Here's how the part is built. I have some questions about the finished solid (model axes, mm). A direction names the side the tool comes from. Round coordinates to 2 decimals unless told otherwise and drop trailing zeros. Loops run counter-clockwise (first coordinate to the right, second up) from the corner with the lowest first, then second, coordinate; pieces in that order, holes last. Notation, with made-up numbers: M -38,-35 L 5,-35 A6 cw 5,-30 Z; hole C -3,52.25 d8. An arc over 180 degrees is marked long. Answer as a JSON object with one key per item and string values.
from build123d import *

# Parameters (mm, degrees)
SKETCH1_W           = 100
SKETCH1_H           = 99
BOSS_EXTRUDE1_DEPTH = 12.75
SKETCH2_W           = 13
SKETCH2_H           = 10
CUT_EXTRUDE1_DEPTH  = 20
LPATTERN1_COUNT     = 5
LPATTERN1_PITCH     = 16
SKETCH3_R           = 1.5
CUT_EXTRUDE2_DEPTH  = 10


with BuildPart() as part:
    # Sketch1 → Boss-Extrude1 (new, symmetric)
    with BuildSketch(Plane(origin=(0, 0, 0), x_dir=(1, 0, 0), z_dir=(0, 1, 0))):
        Rectangle(SKETCH1_W, SKETCH1_H)
    extrude(amount=BOSS_EXTRUDE1_DEPTH, both=True)

    # Sketch2 → Cut-Extrude1 (cut)
    with BuildSketch(Plane.XY.offset(49.5)):
        with Locations((-37, 0)):
            Rectangle(SKETCH2_W, SKETCH2_H)
    cut_extrude1 = extrude(amount=-CUT_EXTRUDE1_DEPTH, mode=Mode.SUBTRACT)

    # LPattern1: Cut-Extrude1 ×5
    with Locations(*[(i * LPATTERN1_PITCH, 0, 0) for i in range(1, LPATTERN1_COUNT)]):
        add(cut_extrude1, mode=Mode.SUBTRACT)

    # Sketch3 → Cut-Extrude2 (cut)
    with BuildSketch(Plane(origin=(0, 0, -49.5), x_dir=(-1, 0, 0), z_dir=(0, 0, -1))):
        with Locations((29, 0)):
            Circle(SKETCH3_R)
    extrude(amount=-CUT_EXTRUDE2_DEPTH, mode=Mode.SUBTRACT)


solid = part.part
Item 1: On a 3-axis mill with a long thin cutter (end or side, diameter ignored), from which of +Z, -Z, +X, -X, +Y, -Y can I reach the whole of each face in a straight line? I mean faces 4 (the face through (-27.5, 0.07, -44.57)), 5 (the face through (-5, 5, 40)), 6 (the face through (-0.7, -5.5, 49.5)). Say none if no direction works.
Resolved:
{"face 4": "-Z", "face 5": "+Z", "face 6": "+Z, +X, -X, +Y, -Y"}
Item 2: I want a section at B-B, the plane x = -17. Please give me the cut outline in (y, z), then the cut area to 3 significant figures.
Resolved:
{"outline": "M -12.75,-49.5 L 12.75,-49.5 L 12.75,49.5 L 5,49.5 L 5,29.5 L -5,29.5 L -5,49.5 L -12.75,49.5 Z", "area": "2,320 mm²"}
Item 3: I'm going to push a flat-ended pin straight in: pin 1 Ø5 at (x, y) = (28.5, 2) entering from +Z. Where does the tip first touch, or does it pass through?
Resolved:
{"pin 1": "z = 29.5"}
Item 4: Please list where these lines run through material, in increasing order: probe 1 along X at (y, z) = (-4.75, 30.5); probe 2 along Y at (x, z) = (-29, -45); probe 3 along Z at (x, y) = (30, -1.75). Write a range as from..to.
Resolved:
{"probe 1": "-50..-43.5, -30.5..-27.5, -14.5..-11.5, 1.5..4.5, 17.5..20.5, 33.5..50", "probe 2": "-12.75..-1.5, 1.5..12.75", "probe 3": "-49.5..29.5"}
Item 5: I want a section at A-A, the plane y = 3. Please give me the cut outline in (x, z), then the cut area to 3 significant figures.
Resolved:
{"outline": "M -50,-49.5 L 50,-49.5 L 50,49.5 L 33.5,49.5 L 33.5,29.5 L 20.5,29.5 L 20.5,49.5 L 17.5,49.5 L 17.5,29.5 L 4.5,29.5 L 4.5,49.5 L 1.5,49.5 L 1.5,29.5 L -11.5,29.5 L -11.5,49.5 L -14.5,49.5 L -14.5,29.5 L -27.5,29.5 L -27.5,49.5 L -30.5,49.5 L -30.5,29.5 L -43.5,29.5 L -43.5,49.5 L -50,49.5 Z", "area": "8,600 mm²"}
Item 6: If we mould it in two halves opening along X, with no side actions, what happens to faces 1 (the face through (-1, 0, -49.5)), 2 (the face through (-37, -5, 40)), 3 (the face through (50, 0, 1))? For each: pulls with the +X half, pulls with the -X half, needs draft (parallel to the pull), parting line crosses it, or undercut.
Resolved:
{"face 1": "needs draft", "face 2": "undercut", "face 3": "pulls with the +X half"}
